Design review of the part built by this model. Coordinates are the model's own, in mm. Coordinates: 2 decimals unless noted, no trailing zeros. Write each loop counter-clockwise with the first axis right and the second up, starting at its lowest first coordinate (ties: lowest second). Pieces come first, ordered by that corner, then holes. Notation, with made-up numbers: (34.25, 40) -> (77.25, 40) arc R35 ccw to (77.25, 77) -> close; hole circle Ø1 at (15, 56). An arc over 180 degrees is marked (long way). Write item = value, one per line. Start each with the question number.
```python
from build123d import *

# Parameters (mm, degrees)
BOSS_EXTRUDE1_DEPTH = 6.35


with BuildPart() as part:
    # Sketch1 → Boss-Extrude1 (new body)
    with BuildSketch(Plane(origin=(120.340372588, -1.499994886, -8.506893725), x_dir=(-0.07052518, -0.000878797, -0.997509612), z_dir=(0.997433673, -0.012432614, -0.070508858))):
        with BuildLine():
            Line((-157.673617622, -825.993121633), (-163.677010897, -824.934561423))
            Line((-163.677010897, -824.934561423), (-168.063361205, -850.003924474))
            Line((-168.063361205, -850.003924474), (-168.063361205, -908.15821278))
            Line((-168.063361205, -908.15821278), (-150.310627761, -908.15821278))
            Line((-150.310627761, -908.15821278), (-150.310627761, -870.05821278))
            ThreePointArc((-150.310627761, -870.05821278), (-145.548127761, -868.782104751), (-140.785627761, -870.05821278))
            Line((-140.785627761, -870.05821278), (-140.785627761, -908.15821278))
            Line((-140.785627761, -908.15821278), (-126.155802929, -908.15821278))
            Line((-126.155802929, -908.15821278), (-126.155802929, -831.550562736))
            Line((-126.155802929, -831.550562736), (-132.159196204, -830.492002526))
            Line((-132.159196204, -830.492002526), (-136.538277842, -855.519822856))
            Line((-136.538277842, -855.519822856), (-162.058583421, -851.054571785))
            Line((-162.058583421, -851.054571785), (-157.673617622, -825.993121633))
        make_face()
        Polygon((-132.159196204, -830.492002526), (-157.673617622, -825.993121633), (-162.058583421, -851.054571785), (-136.538277842, -855.519822856), align=None)
    extrude(amount=BOSS_EXTRUDE1_DEPTH)


solid = part.part
```
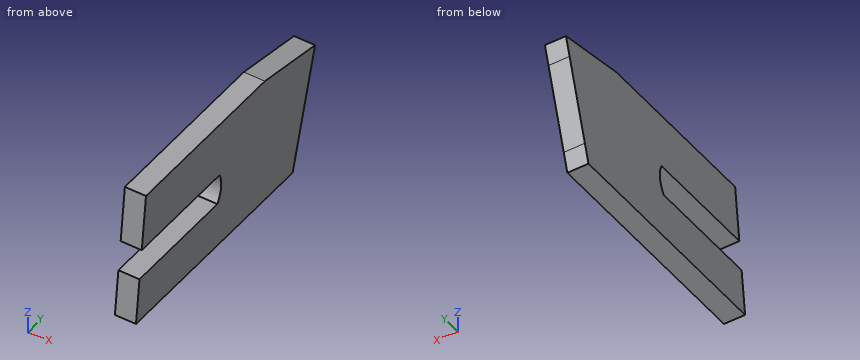
(1) Take a section at C-C, the plane y = -863.5. State the section outline as (x, z) points.
(2) For pin 1 Ø1 at (x, y) = (124.5, -850.5) entering from +Z; pin 2 Ø6 at (x, z) = (123.5, 156.5) entering from -Y; pin 3 Ø4 at (y, z) = (-899.5, 147.5) entering from -X, all flat-tipped, find the tip position at first contact; note any pin that passes through.
(3) Take a section at B-B, the plane z = 127. State the section outline as (x, y) points.
(4) For line 1 (Z direction, x = 122.5, y = -902); line 2 (X direction, y = -851, z = 123); line 3 (Z direction, x = 121.75, y = -887), list the stretches that pass through material, from the lowest coordinate up.
(5) Take a section at A-A, the plane y = -875. State the section outline as (x, z) points, then the cut area to 3 significant figures.
Report:
q1.outline = (118.6, 118.85) -> (124.93, 118.4) -> (127.89, 160.2) -> (121.55, 160.65) -> close
q2.pin_1 = 160.38
q2.pin_2 = -909.52
q2.pin_3 = 120.03
q3.outline = (118.6, -909.47) -> (124.97, -909.55) -> (125.94, -831.42) -> (119.57, -831.42) -> close
q4.line_1 = 118.6 to 133.27, 142.82 to 160.62
q4.line_2 = 119.05 to 125.41
q4.line_3 = 118.64 to 133.31, 142.86 to 160.66
q5.outline = (118.46, 118.87) -> (124.79, 118.42) -> (125.82, 133.01) -> (119.49, 133.46) -> close; (120.16, 142.96) -> (126.49, 142.51) -> (127.75, 160.22) -> (121.41, 160.67) -> close
q5.area = 206 mm2
